from build123d import *


with BuildPart() as part:
    # 草图1 → 旋转9 (revolve)
    with BuildSketch(Plane.XY, mode=Mode.PRIVATE) as revolve_9_sk:
        with BuildLine():
            Line((1.8, -1.45), (2.483096715, -1.45))
            Line((2.483096715, -1.45), (4, -1.469540433))
            Line((4, -1.469540433), (4, -0.6))
            add(Edge.make_bspline(
                [(4, 0.6), (2.330711219, 0), (4, -0.6)],
                knots=[0, 0, 0, 1, 1, 1], degree=2, weights=[1, 2.566282575, 1]))
            Line((4, 0.6), (4, 1.469540433))
            Line((4, 1.469540433), (2.483096715, 1.45))
            Line((2.483096715, 1.45), (1.8, 1.45))
            Line((1.8, 1.45), (1.8, 2.45))
            Line((1.8, 2.45), (1, 2.45))
            Line((1, 2.45), (1, -2.45))
            Line((1, -2.45), (1.8, -2.45))
            Line((1.8, -2.45), (1.8, -1.45))
        make_face()
    revolve(revolve_9_sk.sketch.rotate(Axis((0, 2.07863921, 0), (0, -1, 0)), 90), axis=Axis((0, 2.07863921, 0), (0, -1, 0)))


solid = part.part
Geometry: final body of the model. Coordinates: model frame, mm. A direction names the side the tool comes from. Give positions to 0.01 mm unless a question says otherwise; leave off trailing zeros. Write each loop counter-clockwise with the first axis right and the second up, starting at its lowest first coordinate (ties: lowest second). Pieces come first, ordered by that corner, then holes. Notation, with made-up numbers: (3, -39) - (59, -39) arc R31 cw to (59, -5) - close; hole circle Ø5 at (-38.75, 10.25). An arc over 180 degrees is marked (long way). Return JSON: item names as keys, results as strings. Group by question number.
1) Section A-A on y = 1.7. Return the cut outline in (x, z), plus the area to 3 significant figures.
2) Set-up query: faces 1 (the flat face through (1, -2.45, -1)), 2 (the cylindrical face through (-0.541, -1.943, 1.717)), 3 (the cylindrical face through (-0.541, 1.957, 1.717)). Return all of +Z, -Z, +X, -X, +Y, -Y with unobstructed straight access to the full face (end or side cutting, diameter ignored); none if empty.
3) Line query: line 1 (X direction, y = 1.2, z = 0); line 2 (Y direction, x = 2.25, z = 0.25); line 3 (X direction, y = 0, z = 0). Output: solid intervals per line, ascending.
4) First-contact query: P1, Ø1.5, axis at y = 2, z = 2, coming from the +X side. Flat tip, straight axial feed; report the tip coordinate or a pass-through.
5) Mould query, pull axis Z, two halves, no side actions, for faces 4 (the flat face through (1, 2.45, 1)), 5 (the flat face through (-1, -1.45, -2)), 6 (the cylindrical face through (3.905, 1.041, -0.867)), 7 (the flat face through (-1, 1.45, 2)). Classes: released by +Z, released by -Z, zero draft, split by the parting line, or undercut.
Filled in:
{
 "1": {"outline": "circle Ø3.6 at (0, 0); hole circle Ø2 at (0, 0)", "area": "7.04 mm^2"},
 "2": {"face 1": "+Z, -Z, +X, -X, -Y", "face 2": "-Y", "face 3": "+Y"},
 "3": {"line 1": "x = -4 to -1, 1 to 4", "line 2": "y = -1.45 to 1.45", "line 3": "x = -2.8 to -1, 1 to 2.8"},
 "4": {"P1": "stops at x = 3.72"},
 "5": {"face 4": "zero draft", "face 5": "undercut", "face 6": "split by the parting line", "face 7": "undercut"}
}
